```python
from build123d import *

# Parameters (mm, degrees)
MAIN_DEPTH            = 17.5
SKETCH2_R             = 1.5
SKETCH2_R_2           = 1.25
FIXINGHOLE_DEPTH      = 13
SKETCH3_W             = 12.5
SKETCH3_H             = 23
SERVOSQUAREHOLE_DEPTH = 13
SKETCH4_W             = 5
SKETCH4_H             = 24.5
CABLEHOLE_DEPTH       = 13


with BuildPart() as part:
    # Sketch1 → Main (new body, symmetric)
    with BuildSketch(Plane.XY):
        Polygon((10, 0), (10, 7), (-15, 7), (-15, 0), (-3, 0), (-3, -5), (0, -5), (0, 0), (3.55, 0), (3.55, -1), (6.45, -1), (6.45, 0), align=None)
    extrude(amount=MAIN_DEPTH, both=True)

    # Sketch2 → FixingHole (cut, through all)
    with BuildSketch(Plane(origin=(0, 7, 0), x_dir=(1, 0, 0), z_dir=(0, 1, 0))):
        with Locations((5, 0)):
            Circle(SKETCH2_R)
        with Locations((-6.25, 13.75)):
            Circle(SKETCH2_R_2)
        with Locations((-6.25, -13.75)):
            Circle(SKETCH2_R_2)
    extrude(amount=-FIXINGHOLE_DEPTH, mode=Mode.SUBTRACT)

    # Sketch3 → ServoSquareHole (cut, through all)
    with BuildSketch(Plane(origin=(0, 7, 0), x_dir=(1, 0, 0), z_dir=(0, 1, 0))):
        with Locations((-6.25, 0)):
            Rectangle(SKETCH3_W, SKETCH3_H)
    extrude(amount=-SERVOSQUAREHOLE_DEPTH, mode=Mode.SUBTRACT)

    # Sketch4 → CableHole (cut, through all)
    with BuildSketch(Plane(origin=(0, 7, 0), x_dir=(1, 0, 0), z_dir=(0, 1, 0))):
        with Locations((-6.25, 0)):
            Rectangle(SKETCH4_W, SKETCH4_H)
    extrude(amount=-CABLEHOLE_DEPTH, mode=Mode.SUBTRACT)


solid = part.part
```
Verification items for the finished model (mm, model axes). A direction names the side the tool comes from. Coordinates: 2 decimals unless noted, no trailing zeros. Write each loop counter-clockwise with the first axis right and the second up, starting at its lowest first coordinate (ties: lowest second). Pieces come first, ordered by that corner, then holes. Notation, with made-up numbers: M 51,20.25 L 88,20.25 A27 ccw 88,52.25 Z; hole C -16,21.5 d9. An arc over 180 degrees is marked long. One line per item, written item: value.
Item 1: Section check D-D, the plane x = -6.25. Record the boundary of the cut face in (y, z), plus the area to 3 significant figures.
Check sheet entries:
outline: M 0,-17.5 L 7,-17.5 L 7,-15 L 0,-15 Z; M 0,-12.5 L 7,-12.5 L 7,-12.25 L 0,-12.25 Z; M 0,12.25 L 7,12.25 L 7,12.5 L 0,12.5 Z; M 0,15 L 7,15 L 7,17.5 L 0,17.5 Z
area: 38.5 mm^2
Item 2: Mould release check, pull along Z, two halves, no side actions. Record for faces 4 (the flat face through (5, -1, -9)), 5 (the flat face through (-2, 1, -11.5)), 6 (the flat face through (-3, 4, 17.5)): pulls with the +Z half, pulls with the -Z half, needs draft (parallel to the pull), parting line crosses it, or undercut.
Check sheet entries:
face 4: needs draft
face 5: undercut
face 6: pulls with the +Z half
Item 3: Scan lines: line 1 along X through (y, z) = (4.5, 0); line 2 along Z through (x, y) = (-6.25, 4.75); line 3 along X through (y, z) = (4.5, 10.5). Record each from-to range of solid material in increasing order.
Check sheet entries:
line 1: x = -15 to -12.5, 0 to 3.5, 6.5 to 10
line 2: z = -17.5 to -15, -12.5 to -12.25, 12.25 to 12.5, 15 to 17.5
line 3: x = -15 to -12.5, 0 to 10
Item 4: Access from +Z, -Z, +X, -X, +Y, -Y to the whole of each face (thin tool, end or side, straight path). Record for faces 1 (the flat face through (3.55, -0.5, 9.1)), 2 (the flat face through (0, 4, 0)), 3 (the flat face through (5, -1, 9)).
Check sheet entries:
face 1: +Z, -Z, -Y
face 2: +Y, -Y
face 3: +Z, -Z, +X, -Y
Item 5: Section check C-C, the plane x = 5. Record the boundary of the cut face in (y, z).
Check sheet entries:
outline: M -1,-17.5 L 7,-17.5 L 7,-1.5 L -1,-1.5 Z; M -1,1.5 L 7,1.5 L 7,17.5 L -1,17.5 Z
Item 6: Gauge pin test, flat ends, axial feed: pin 1 Ø1 at (y, z) = (-2, -7.5) entering from +X; pin 2 Ø2.5 at (x, z) = (5.5, -11) entering from -Y; pin 3 Ø1.8 at (x, z) = (2.5, -0.5) entering from -Y; pin 4 Ø2.5 at (y, z) = (-1.5, 13.5) entering from -X. Record the tip position at first contact, or that the pin passes through.
Check sheet entries:
pin 1: passes through
pin 2: stops at y = -1
pin 3: stops at y = 0
pin 4: stops at x = -3
Item 7: Section check B-B, the plane y = -3.75. Record the boundary of the cut face in (x, z), plus the area to 3 significant figures.
Check sheet entries:
outline: M -3,-17.5 L 0,-17.5 L 0,-11.5 L -3,-11.5 Z; M -3,11.5 L 0,11.5 L 0,17.5 L -3,17.5 Z
area: 36.0 mm^2
Item 8: Section check A-A, the plane z = 6. Record the boundary of the cut face in (x, y), plus the area to 3 significant figures.
Check sheet entries:
outline: M -15,0 L -12.5,0 L -12.5,7 L -15,7 Z; M 0,0 L 3.55,0 L 3.55,-1 L 6.45,-1 L 6.45,0 L 10,0 L 10,7 L 0,7 Z
area: 90.4 mm^2
